Drawing for the job (mm, zero at the part's lowest x, y, z). Round coordinates to 2 decimals unless told otherwise and drop trailing zeros. Order: outer loops, then holes, each group sorted by start corner. A loop starts at its lowest first (then second) coordinate and runs counter-clockwise, first axis right, second up. Notation, with made-up numbers: (74, -40) -> (94, -40) arc R37 ccw to (94, -1) -> close; hole circle Ø4 at (57, -34.5). An arc over 180 degrees is marked (long way). Answer as CSV lines item,"result". Start each with the question number.
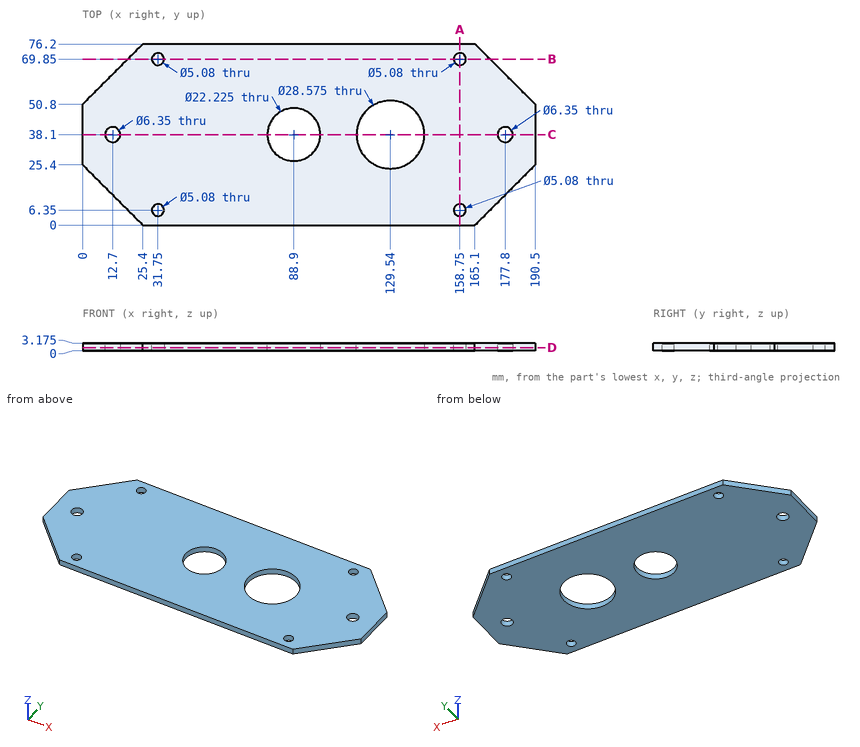
Q1. Slice it at C-C, the plane y = 38.1. Write the cut outline in (x, z) (1 decimal), plus the area to 3 significant figures.
Q2. Slice it at B-B, the plane y = 69.85. Write the cut outline in (x, z) (3 decimals).
Q3. Slice it at D-D, the plane z = 1.25. Count the separate pieces of the cut face and the enclosed holes in it, plus the area to 3 significant figures.
Q4. Slice it at A-A, the plane x = 158.75. Write the cut outline in (y, z) (3 decimals), plus the area to 3 significant figures.
Q5. Probe L1, parallel to X at y = 68, z = 1.75; L2, parallel to X at y = 40.5, z = 2.35; L3, parallel to X at y = 34, z = 2.3. List the from-to ranges inside material, lowest first.
Q6. Flat gauge pins, fed straight in: pin 1 Ø8.5 at (x, y) = (177.8, 38.1) entering from +Z (3 decimals); pin 2 Ø23 at (x, y) = (129.54, 38.1) entering from -Z; pin 3 Ø1 at (y, z) = (61.5, 2.5) entering from -X. Where does each tip first touch, or does it go through?
Solutions:
1,outline,"(0, 0) -> (9.5, 0) -> (9.5, 3.2) -> (0, 3.2) -> close; (15.9, 0) -> (77.8, 0) -> (77.8, 3.2) -> (15.9, 3.2) -> close; (100, 0) -> (115.3, 0) -> (115.3, 3.2) -> (100, 3.2) -> close; (143.8, 0) -> (174.6, 0) -> (174.6, 3.2) -> (143.8, 3.2) -> close; (181, 0) -> (190.5, 0) -> (190.5, 3.2) -> (181, 3.2) -> close"
1,area,"403 mm2"
2,outline,"(19.05, 0) -> (29.21, 0) -> (29.21, 3.175) -> (19.05, 3.175) -> close; (34.29, 0) -> (156.21, 0) -> (156.21, 3.175) -> (34.29, 3.175) -> close; (161.29, 0) -> (171.45, 0) -> (171.45, 3.175) -> (161.29, 3.175) -> close"
3,separate pieces,"1"
3,enclosed holes,"8"
3,area,"12,100 mm2"
4,outline,"(0, 0) -> (3.81, 0) -> (3.81, 3.175) -> (0, 3.175) -> close; (8.89, 0) -> (67.31, 0) -> (67.31, 3.175) -> (8.89, 3.175) -> close; (72.39, 0) -> (76.2, 0) -> (76.2, 3.175) -> (72.39, 3.175) -> close"
4,area,"210 mm2"
5,L1,"x = 17.2 to 30.01, 33.49 to 157.01, 160.49 to 173.3"
5,L2,"x = 0 to 10.62, 14.78 to 78.05, 99.75 to 115.46, 143.62 to 175.72, 179.88 to 190.5"
5,L3,"x = 0 to 78.57, 99.23 to 115.85, 143.23 to 190.5"
6,pin 1,"stops at z = 3.175"
6,pin 2,"passes through"
6,pin 3,"stops at x = 10.2"
